Part model, mm, in its own coordinate system. A direction names the side the tool comes from. Round coordinates to 2 decimals unless told otherwise and drop trailing zeros. Loops run counter-clockwise (first coordinate to the right, second up) from the corner with the lowest first, then second, coordinate; pieces in that order, holes last.
(1) Mould opens along Y. For faces 1 (the face through (-2, 0, 2.032)), 2 (the face through (12.7, 0, 0)), 3 (the face through (6.06, -0.69, -3.1)) say: +Y half, -Y half, draft (parallel to the pull), parting line (faces both ways), or undercut.
(2) Flat gauge pins, fed straight in: pin 1 (2.5 mm diameter, centred on x = -2, y = -0.5, fed in from +Z); pin 2 (6.5 mm diameter, centred on y = -0.5, z = -3, fed in from +X); pin 3 (6 mm diameter, centred on x = 5.5, y = -3.5, fed in from +Z); pin 4 (1.5 mm diameter, centred on y = 4, z = -2, fed in from +X). Where does each tip first touch, or does it go through?
(3) Probe probe 1 along X at (y, z) = (-0.75, 1.75); probe 2 along X at (y, z) = (1, -3.75); probe 3 along Z at (x, y) = (0.5, -1). List the from-to ranges inside material, lowest first.
(4) Cut at A-A on x = 3.5. List the corners of the cut face in (y, z) (3 decimals).
(5) Tool access for faces 4 (the face through (-0.3, 6.1, -2.53)), 5 (the face through (0, -2, -3)), 6 (the face through (-1.92, -1.77, -1)): list every direction of +Z, -Z, +X, -X, +Y, -Y with a clear straight run to the whole face (end or side of a thin tool).
Autodesk Inventor part; units mm, degrees
ref_plane "screw_XY" through (0, 0, 0) normal (1, 0, 0) x (0, 0, -1)
ref_plane "screw_YZ" through (0, 0, 0) normal (0, 0, -1) x (0, 1, 0)
ref_plane "screw_ZX" through (0, 0, 0) normal (0, 1, 0) x (1, 0, 0)
sketch "Sketch_1" plane through (0, 0, 0) normal (0, 0, 1) x (1, 0, 0)
  line L0 (12.7, 0) -> (-3.048, 0)
  line L1 (-3.048, 0) -> (-3.048, 2.4384)
  arc A0 (-0.6096, 5.9436) -> (-3.048, 2.4384) centre (3.3013, 0.6222) ccw
  line L2 (-0.6096, 5.9436) -> (-0.6096, 6.604)
  line L3 (-0.6096, 6.604) -> (0, 6.604)
  line L4 (0, 6.604) -> (0, 3.175)
  line L5 (0, 3.175) -> (11.9444, 3.175)
  line L6 (11.9444, 3.175) -> (12.7, 2.4194)
  line L7 (12.7, 2.4194) -> (12.7, 0)
  line L8 (12.7, 0) -> (-3.048, 0)
revolve "Revolution1" add sketch "Sketch_1" angle 360 about axis through (12.7, 0, 0) along (1, 0, 0)
thread "Thread1"
sketch "Sketch_2" plane through (-3.048, 0, 0) normal (1, 0, 0) x (0, 0, -1)
  line L0 (-2.032, -1.1732) -> (0, -2.3464)
  line L1 (0, -2.3464) -> (2.032, -1.1732)
  line L2 (2.032, -1.1732) -> (2.032, 1.1732)
  line L3 (2.032, 1.1732) -> (0, 2.3464)
  line L4 (0, 2.3464) -> (-2.032, 1.1732)
  line L5 (-2.032, 1.1732) -> (-2.032, -1.1732)
extrude "Extrusion1" cut sketch "Sketch_2" along normal blind 2.286
ref_plane "screw_XY" through (0, 0, 0) normal (1, 0, 0) x (0, 0, -1)
ref_plane "screw_YZ" through (0, 0, 0) normal (0, 0, -1) x (0, 1, 0)
ref_plane "screw_ZX" through (0, 0, 0) normal (0, 1, 0) x (1, 0, 0)
ref_plane "to_nut_XY" through (12.7, 0, 0) normal (1, 0, 0) x (0, 0, -1)
ref_plane "to_nut_YZ" through (12.7, 0, 0) normal (0, 0, -1) x (0, 1, 0)
ref_plane "to_nut_ZX" through (12.7, 0, 0) normal (0, 1, 0) x (1, 0, 0)
properties part number "3342"
Final values:
1. face 1: undercut
1. face 2: draft
1. face 3: parting line
2. pin 1: stops at z = 5.82
2. pin 2: stops at x = 12.7
2. pin 3: stops at z = 3.14
2. pin 4: stops at x = 0
3. probe 1: x = -0.76 to 12.7
3. probe 2: x = -2.44 to 0
3. probe 3: z = -3.01 to 3.01
4. outline: circle Ø6.35 at (0, 0)
5. face 4: +X, -X
5. face 5: +X
5. face 6: -X
